Verification items for the finished model (mm, model axes). Face numbers are marked on the shaded views. A direction names the side the tool comes from. Coordinates: 2 decimals unless noted, no trailing zeros. Write each loop counter-clockwise with the first axis right and the second up, starting at its lowest first coordinate (ties: lowest second). Pieces come first, ordered by that corner, then holes. Notation, with made-up numbers: (39.5, 41.5) - (56.5, 41.5) arc R26 ccw to (56.5, 79.5) - close; hole circle Ø5 at (55, 42.5). An arc over 180 degrees is marked (long way). Use CSV: the item, a comma, the result in double quotes. Start each with the question number.
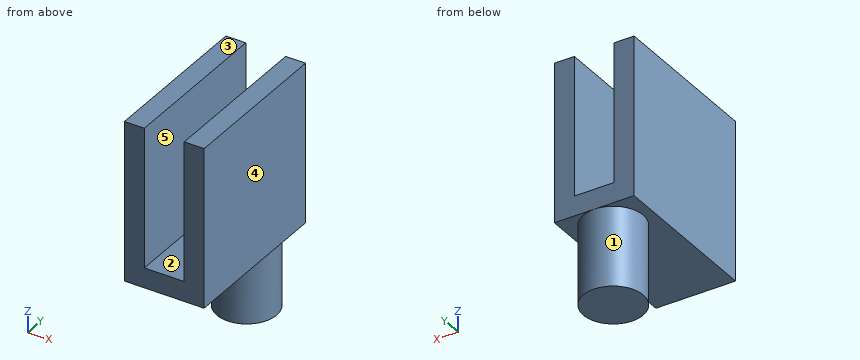
Autodesk Inventor part; units mm, degrees
ref_plane "YZ Plane" through (0, 0, 0) normal (1, 0, 0) x (0, 1, 0)
ref_plane "XZ Plane" through (0, 0, 0) normal (0, 1, 0) x (-1, 0, 0)
ref_plane "XY Plane" through (0, 0, 0) normal (0, 0, 1) x (1, 0, 0)
sketch "Body_Skt" plane through (0, 0, 0) normal (0, 0, 1) x (1, 0, 0)
  line L0 (-2, -4) -> (2, -4)
  line L1 (2, -4) -> (2, 4)
  line L2 (2, 4) -> (-2, 4)
  line L3 (-2, 4) -> (-2, -4)
  line L4 (-2, -4) -> (2, 4) construction
  line L5 (2, -4) -> (-2, 4) construction
  point P0 (0, 0)
  dimension "d0" = 4
  dimension "d1" = 8
extrude "Body" add sketch "Body_Skt" along normal blind 8
sketch "Wall_Skt" plane through (-2, -4, 0) normal (0, -1, 0) x (1, 0, 0)
  line L0 (0, 8) -> (4, 8)
  line L1 (3, 8) -> (1, 8)
  line L2 (1, 8) -> (1, 1)
  line L3 (1, 1) -> (3, 1)
  line L4 (3, 1) -> (3, 8)
  line L5 (4, 0) -> (4, 8)
  line L6 (0, 0) -> (4, 0)
  line L7 (0, 0) -> (0, 8)
  point P0 (2, 0)
  dimension "d4" = 1
  dimension "d5" = 1
  dimension "d6" = 1
extrude "Wall" cut sketch "Wall_Skt" against normal through all contours L0 L4 L3 L2
sketch "Leg_Skt" plane through (0, 0, 0) normal (0, 0, -1) x (-1, 0, 0)
  circle A0 centre (0, 2.5) radius 1.5
  line L0 (-2, 4) -> (2, 4)
  line L1 (0, 0) -> (0, 4) construction
  dimension "d10" = 3
extrude "Leg" add sketch "Leg_Skt" along normal blind 4
equation "\"d0\" = wall_inner_diam + 2 * wall_outer_diam"
equation "\"d1\" = wall_widh"
equation "\"d2\" = wall_height"
equation "\"d4\" = wall_outer_diam"
equation "\"d5\" = wall_outer_diam"
equation "\"d6\" = wall_outer_diam"
equation "\"d7\" = d1 - wall_outer_diam"
equation "\"d10\" = leg_diam"
equation "\"d11\" = leg_height"
equation "\"wall_inner_diam\" = 2"
equation "\"wall_outer_diam\" = 1"
equation "\"wall_height\" = 8"
equation "\"leg_diam\" = 3"
equation "\"leg_height\" = 4"
equation "\"wall_widh\" = 8"
properties part number "coffee"
Q1. Scan lines: line 1 along X through (y, z) = (-1.75, 3); line 2 along Z through (x, y) = (-0.35, 2.75); line 3 along Z through (x, y) = (-1.05, 1). Record each from-to range of solid material in increasing order. Write a range as from..to.
Q2. Cross-section at D-D (y = 2.5). Record the cut outline in (x, z), plus the area to 3 significant figures.
Q3. Cross-section at A-A (z = 6.5). Record the cut outline in (x, y).
Q4. Cross-section at C-C (y = -1.25). Record the cut outline in (x, z), plus the area to 3 significant figures.
Q5. Tool access check on the marked faces 4 and 5. Record the directions out of +Z, -Z, +X, -X, +Y, -Y that give a thin tool (end or side, any length) a straight path to the whole face; none if there is none.
Q6. Cross-section at B-B (x = 1.2). Record the cut outline in (y, z), plus the area to 3 significant figures.
Q7. Release check for a two-part mould opening along X. For the marked faces 1, 2 and 3 record: released by +X, released by -X, zero draft, split by the parting line, or undercut.
Q8. Gauge pin test, flat end, axial feed: pin 1 (1.6 mm diameter, centred on x = 0, y = -1, fed in from +Z). Record the tip position at first contact, or that the pin passes through.
Reply:
1,line 1,"-2..-1, 1..2"
1,line 2,"-4..1"
1,line 3,"0..8"
2,outline,"(-2, 0) - (-1.5, 0) - (-1.5, -4) - (1.5, -4) - (1.5, 0) - (2, 0) - (2, 8) - (1, 8) - (1, 1) - (-1, 1) - (-1, 8) - (-2, 8) - close"
2,area,"30.0 mm^2"
3,outline,"(-2, -4) - (-1, -4) - (-1, 4) - (-2, 4) - close; (1, -4) - (2, -4) - (2, 4) - (1, 4) - close"
4,outline,"(-2, 0) - (2, 0) - (2, 8) - (1, 8) - (1, 1) - (-1, 1) - (-1, 8) - (-2, 8) - close"
4,area,"18.0 mm^2"
5,face 4,"+Z, -Z, +X, +Y, -Y"
5,face 5,"+Z, +Y, -Y"
6,outline,"(-4, 0) - (1.6, 0) - (1.6, -4) - (3.4, -4) - (3.4, 0) - (4, 0) - (4, 8) - (-4, 8) - close"
6,area,"71.2 mm^2"
7,face 1,"split by the parting line"
7,face 2,"undercut"
7,face 3,"zero draft"
8,pin 1,"z = 1"
